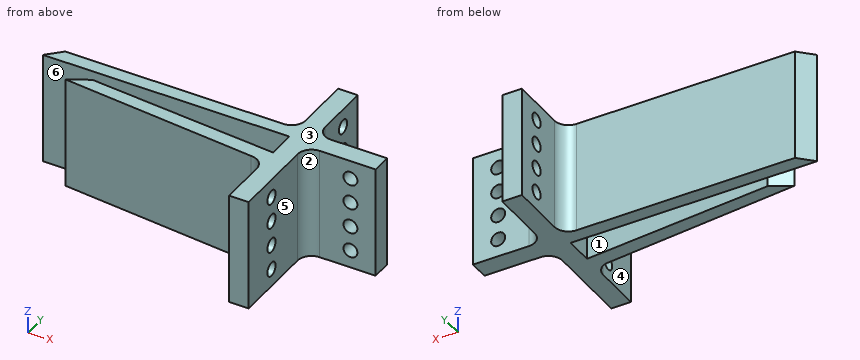
```python
from build123d import *

# Parameters (mm, degrees)
PAD_DEPTH              = 40
SKETCH001_R            = 2.5
POCKET_DEPTH           = 7
LINEARPATTERN_COUNT    = 4
LINEARPATTERN_PITCH    = 9
SKETCH002_R            = 2.5
POCKET001_DEPTH        = 7
LINEARPATTERN001_COUNT = 4
LINEARPATTERN001_PITCH = 9
SKETCH003_R            = 2.5
POCKET002_DEPTH        = 7
LINEARPATTERN002_COUNT = 4
LINEARPATTERN002_PITCH = 9


with BuildPart() as part:
    # Sketch → Pad (new body)
    with BuildSketch(Plane.XY):
        with BuildLine():
            Line((-7, 0), (0, 0))
            Line((0, 0), (0, 30))
            ThreePointArc((5.000001, 35), (1.464466, 33.535534), (0, 30))
            Line((5.000001, 35), (25, 35))
            Line((25, 35), (25, 42))
            Line((25, 42), (5, 42))
            ThreePointArc((0, 47), (1.464466, 43.464466), (5, 42))
            Line((0, 47), (0, 67))
            Line((0, 67), (-7, 67))
            Line((-7, 67), (-7, 47))
            ThreePointArc((-12, 42), (-8.464466, 43.464466), (-7, 47))
            Line((-12, 42), (-90, 42))
            Line((-90, 42), (-95, 37))
            Line((-95, 37), (-7, 37))
            Line((-7, 37), (-7, 27))
            Line((-7, 27), (-75, 33))
            Line((-75, 33), (-82.351578, 29))
            Line((-82.351578, 29), (-12, 22))
            ThreePointArc((-7, 17), (-8.464466, 20.535534), (-12, 22))
            Line((-7, 17), (-7, 0))
        make_face()
    extrude(amount=PAD_DEPTH)

    # Sketch001 → Pocket (cut)
    with BuildSketch(Plane.YZ):
        with Locations((58, 33.523144)):
            Circle(SKETCH001_R)
    pocket = extrude(amount=-POCKET_DEPTH, mode=Mode.SUBTRACT)

    # LinearPattern: Pocket ×4
    with Locations(*[(0, 0, -i * LINEARPATTERN_PITCH) for i in range(1, LINEARPATTERN_COUNT)]):
        add(pocket, mode=Mode.SUBTRACT)

    # Sketch002 → Pocket001 (cut)
    with BuildSketch(Plane.XZ.offset(-35)):
        with Locations((16, 33.395916)):
            Circle(SKETCH002_R)
    pocket001 = extrude(amount=-POCKET001_DEPTH, mode=Mode.SUBTRACT)

    # LinearPattern001: Pocket001 ×4
    with Locations(*[(0, 0, -i * LINEARPATTERN001_PITCH) for i in range(1, LINEARPATTERN001_COUNT)]):
        add(pocket001, mode=Mode.SUBTRACT)

    # Sketch003 → Pocket002 (cut)
    with BuildSketch(Plane.YZ):
        with Locations((14, 33.378235)):
            Circle(SKETCH003_R)
    pocket002 = extrude(amount=-POCKET002_DEPTH, mode=Mode.SUBTRACT)

    # LinearPattern002: Pocket002 ×4
    with Locations(*[(0, 0, -i * LINEARPATTERN002_PITCH) for i in range(1, LINEARPATTERN002_COUNT)]):
        add(pocket002, mode=Mode.SUBTRACT)


solid = part.part
```
Model file for the job. Use its own axes, mm. Face numbers are marked on the shaded views. A direction names the side the tool comes from. Give positions to 0.01 mm unless a question says otherwise; leave off trailing zeros. Loops run counter-clockwise (first coordinate to the right, second up) from the corner with the lowest first, then second, coordinate; pieces in that order, holes last. Notation, with made-up numbers: (33, 59.5) -> (74, 59.5) arc R16 cw to (74, 71.5) -> close; hole circle Ø6 at (39.25, 38). An arc over 180 degrees is marked (long way). Write each question's results on one line, items separated by ' | '.
(1) Tool access for the marked faces 4, 5 and 6: list every direction of +Z, -Z, +X, -X, +Y, -Y with a clear straight run to the whole face (end or side of a thin tool).
Geometry results:
face 4: +Z, -Z, -X, -Y | face 5: +Z, -Z, +X, -Y | face 6: +Z, -Z, -X
(2) Cut at C-C on z = 28.5. List the corners of the cut face in (x, y).
Geometry results:
outline: (-95, 37) -> (-7, 37) -> (-7, 27) -> (-75, 33) -> (-82.35, 29) -> (-12, 22) arc R5 cw to (-7, 17) -> (-7, 0) -> (0, 0) -> (0, 30) arc R5 cw to (5, 35) -> (25, 35) -> (25, 42) -> (5, 42) arc R5 cw to (0, 47) -> (0, 67) -> (-7, 67) -> (-7, 47) arc R5 cw to (-12, 42) -> (-90, 42) -> close
(3) Probe line 1 along Z through (x, y) = (-5, 58); line 2 along Z through (x, y) = (16, 37); line 3 along Y through (x, z) = (-89.5, 6.5). List the from-to ranges inside material, lowest first.
Geometry results:
line 1: z = 0 to 4.02, 9.02 to 13.02, 18.02 to 22.02, 27.02 to 31.02, 36.02 to 40 | line 2: z = 0 to 3.9, 8.9 to 12.9, 17.9 to 21.9, 26.9 to 30.9, 35.9 to 40 | line 3: y = 37 to 42
(4) Cut at B-B on x = 16. List the corners of the cut face in (y, z).
Geometry results:
outline: (35, 0) -> (42, 0) -> (42, 3.9) -> (35, 3.9) -> close; (35, 8.9) -> (42, 8.9) -> (42, 12.9) -> (35, 12.9) -> close; (35, 17.9) -> (42, 17.9) -> (42, 21.9) -> (35, 21.9) -> close; (35, 26.9) -> (42, 26.9) -> (42, 30.9) -> (35, 30.9) -> close; (35, 35.9) -> (42, 35.9) -> (42, 40) -> (35, 40) -> close
(5) Pull direction Y, two halves, no side cores. Call the marked faces 1, 2 and 3: released by +Y, released by -Y, zero draft, split by the parting line, or undercut.
Geometry results:
face 1: undercut | face 2: released by -Y | face 3: zero draft
(6) Flat gauge pins, fed straight in: pin 1 Ø8 at (x, z) = (16, 15.4) entering from -Y; pin 2 Ø18.5 at (y, z) = (7.5, 26.5) entering from -X; pin 3 Ø3 at (x, z) = (-1, 33.5) entering from -Y; pin 4 Ø1 at (x, z) = (-30, 4.5) entering from +Y. Where does each tip first touch, or does it go through?
Geometry results:
pin 1: stops at y = 35 | pin 2: stops at x = -7 | pin 3: stops at y = 0 | pin 4: stops at y = 42
(7) Cut at D-D on x = -3.5. Give the number of separate pieces and of enclosed holes in the cut face, and give its area (3 significant figures).
Geometry results:
separate pieces: 1 | enclosed holes: 8 | area: 2,520 mm²
(8) Cut at A-A on y = 58. List the corners of the cut face in (x, z), and give its area (3 significant figures).
Geometry results:
outline: (-7, 0) -> (0, 0) -> (0, 4.02) -> (-7, 4.02) -> close; (-7, 9.02) -> (0, 9.02) -> (0, 13.02) -> (-7, 13.02) -> close; (-7, 18.02) -> (0, 18.02) -> (0, 22.02) -> (-7, 22.02) -> close; (-7, 27.02) -> (0, 27.02) -> (0, 31.02) -> (-7, 31.02) -> close; (-7, 36.02) -> (0, 36.02) -> (0, 40) -> (-7, 40) -> close | area: 140 mm²
